Can you work these out from the model? Positions are in its coordinate system, mm. A direction names the side the tool comes from. Coordinates: 2 decimals unless noted, no trailing zeros. Order: outer loops, then holes, each group sorted by start corner. A loop starts at its lowest first (then second) coordinate and runs counter-clockwise, first axis right, second up.
```python
from build123d import *

# Parameters (mm, degrees)
SKETCH_1_W          = 42.5
SKETCH_1_H          = 42.5
EXTRUDE_1_DEPTH     = 59.15
SKETCH_2_R          = 10
EXTRUDE_2_DEPTH     = 3
SKETCH_3_R          = 4
EXTRUDE_3_DEPTH     = 20
HOLE_WIZARD_3_D     = 3.3
HOLE_WIZARD_3_DEPTH = 11.5
HOLE_WIZARD_3_TIP   = 0.991420021
EXTRUDE_4_DEPTH     = 12


with BuildPart() as part:
    # 스케치1 → 돌출1 (new body)
    with BuildSketch(Plane(origin=(0, 0, 0), x_dir=(-1, 0, 0), z_dir=(0, 1, 0))):
        with Locations((21.25, -21.25)):
            Rectangle(SKETCH_1_W, SKETCH_1_H)
    extrude(amount=EXTRUDE_1_DEPTH)

    # 스케치2 → 돌출2 (add)
    with BuildSketch(Plane(origin=(0, 59.15, 0), x_dir=(-1, 0, 0), z_dir=(0, 1, 0))):
        with Locations((21.25, -21.25)):
            Circle(SKETCH_2_R)
    extrude(amount=EXTRUDE_2_DEPTH)

    # 스케치3 → 돌출3 (add)
    with BuildSketch(Plane(origin=(0, 62.15, 0), x_dir=(-1, 0, 0), z_dir=(0, 1, 0))):
        with Locations((21.25, -21.25)):
            Circle(SKETCH_3_R)
    extrude(amount=EXTRUDE_3_DEPTH)

    # 구멍3
    with Locations(Plane(origin=(0, 59.15, 0), x_dir=(1, 0, 0), z_dir=(0, 1, 0))):
        with Locations((-4.25, 38.25), (-4.25, 4.25), (-38.25, 4.25), (-38.25, 38.25)):
            Hole(HOLE_WIZARD_3_D / 2, depth=HOLE_WIZARD_3_DEPTH)
            with Locations((0, 0, -(HOLE_WIZARD_3_DEPTH + HOLE_WIZARD_3_TIP / 2))):  # 118° drill point
                Cone(0, HOLE_WIZARD_3_D / 2, HOLE_WIZARD_3_TIP, mode=Mode.SUBTRACT)

    # 스케치6 → 돌출4 (cut)
    with BuildSketch(Plane(origin=(0, 82.15, 0), x_dir=(-1, 0, 0), z_dir=(0, 1, 0))):
        with BuildLine():
            Line((24.75, -19.313508327), (24.75, -23.186491673))
            ThreePointArc((24.75, -23.186491673), (25.25, -21.25), (24.75, -19.313508327))
        make_face()
    extrude(amount=-EXTRUDE_4_DEPTH, mode=Mode.SUBTRACT)


solid = part.part
```
1. Please list where these lines run through material, in increasing order: probe 1 along Z at (x, y) = (-38.25, 55.25); probe 2 along X at (y, z) = (50, -4); probe 3 along Y at (x, z) = (-25.5, -19.5).
Completed:
probe 1: z = -42.5 to -39.9, -36.6 to -5.9, -2.6 to 0
probe 2: x = -42.5 to -39.88, -36.62 to -5.88, -2.62 to 0
probe 3: y = 0 to 62.15
2. Imagine slicing it at A-A on y = 50.5. Please give me the cut outline in (x, z).
Completed:
outline: (-42.5, -42.5) - (0, -42.5) - (0, 0) - (-42.5, 0) - close; hole circle Ø3.3 at (-38.25, -38.25); hole circle Ø3.3 at (-38.25, -4.25); hole circle Ø3.3 at (-4.25, -38.25); hole circle Ø3.3 at (-4.25, -4.25)
3. Imagine slicing it at D-D on x = -8.5. Please give me the cut outline in (y, z), then the cut area to 3 significant figures.
Completed:
outline: (0, -42.5) - (59.15, -42.5) - (59.15, 0) - (0, 0) - close
area: 2,510 mm2
4. I'm going to push flat-ended pins straight in: pin 1 (2 mm diameter, centred on x = -31.5, z = -12, fed in from +Y); pin 2 (4.5 mm diameter, centred on y = 74, z = -21, fed in from -X); pin 3 (10 mm diameter, centred on x = -23, y = 71.5, fed in from -Z). Where does each tip first touch, or does it pass through?
Completed:
pin 1: stops at y = 59.15
pin 2: stops at x = -24.75
pin 3: stops at z = -25.25
5. Imagine slicing it at C-C on z = -21.25. Please give me the cut outline in (x, y).
Completed:
outline: (-42.5, 0) - (0, 0) - (0, 59.15) - (-11.25, 59.15) - (-11.25, 62.15) - (-17.25, 62.15) - (-17.25, 82.15) - (-24.75, 82.15) - (-24.75, 70.15) - (-25.25, 70.15) - (-25.25, 62.15) - (-31.25, 62.15) - (-31.25, 59.15) - (-42.5, 59.15) - close
6. Thinking about a two-plate mould opening in X: for faces 4 (the cylindrical face through (-3.034, 53.32, -39.365)), 5 (the cylindrical face through (-17.254, 72.01, -21.074)), 6 (the flat face through (-12, 59.15, -16)), which applies, pulls with the +X half, pulls with the -X half, needs draft (parallel to the pull), parting line crosses it, or undercut?
Completed:
face 4: undercut
face 5: parting line crosses it
face 6: needs draft
7. Imagine slicing it at B-B on x = -21.25. Please give me the cut outline in (y, z).
Completed:
outline: (0, -42.5) - (59.15, -42.5) - (59.15, -31.25) - (62.15, -31.25) - (62.15, -25.25) - (82.15, -25.25) - (82.15, -17.25) - (62.15, -17.25) - (62.15, -11.25) - (59.15, -11.25) - (59.15, 0) - (0, 0) - close
8. On a 3-axis mill with a long thin cutter (end or side, diameter ignored), from which of +Z, -Z, +X, -X, +Y, -Y can I reach the whole of each face in a straight line? I mean faces 1 (the flat face through (-24.75, 76, -21)), 2 (the flat face through (-21, 0, -21)), 3 (the cylindrical face through (-30.79, 60.63, -18.25)). Say none if no direction works.
Completed:
face 1: +Z, -Z, -X, +Y
face 2: +Z, -Z, +X, -X, -Y
face 3: +Y
